CAD build for the part. Positions are in the model's coordinates, mm. A direction names the side the tool comes from. Round coordinates to 2 decimals unless told otherwise and drop trailing zeros. Loops run counter-clockwise (first coordinate to the right, second up) from the corner with the lowest first, then second, coordinate; pieces in that order, holes last. Notation, with made-up numbers: (82, -39) - (131, -39) arc R13 ccw to (131, -34) - close; hole circle Ø7 at (-14.5, 39.5). An arc over 180 degrees is marked (long way). Use one line per item in the form item = value.
from build123d import *

# Parameters (mm, degrees)
SKETCH2_R           = 2.286
BOSS_EXTRUDE1_DEPTH = 5.08
FILLET1_R           = 2.54
FILLET2_R           = 0.635
SKETCH3_W           = 3.81
SKETCH3_H           = 1.905
CUT_EXTRUDE1_DEPTH  = 6.08


with BuildPart() as part:
    # Sketch2 → Boss-Extrude1 (new body)
    with BuildSketch(Plane.XY):
        with BuildLine():
            ThreePointArc((20.32, -7.62), (9.895271997, -11.792143987), (-1.27, -12.983127033))
            Line((-1.27, -12.983127033), (-1.27, -3.81))
            Line((-1.27, -3.81), (20.32, -3.81))
            Line((20.32, -3.81), (20.32, 3.81))
            Line((20.32, 3.81), (-5.08, 3.81))
            Line((-5.08, 3.81), (-5.08, -19.05))
            Line((-5.08, -19.05), (20.32, -19.05))
            Line((20.32, -19.05), (20.32, -7.62))
        make_face()
        Circle(SKETCH2_R, mode=Mode.SUBTRACT)
    extrude(amount=BOSS_EXTRUDE1_DEPTH)

    # Fillet1
    fillet1_edges = [part.edges().sort_by_distance(p)[0] for p in [
        (-5.08, 3.81, 2.54),
        (20.32, 3.81, 2.54),
        (20.32, -3.81, 2.54),
        (-1.27, -3.81, 2.54),
        (20.32, -19.05, 2.54),
        (-5.08, -19.05, 2.54),
    ]]
    fillet(fillet1_edges, radius=FILLET1_R)

    # Fillet2
    fillet2_edges = [part.edges().sort_by_distance(p)[0] for p in [
        (20.32, -7.62, 2.54),
    ]]
    fillet(fillet2_edges, radius=FILLET2_R)

    # Sketch3 → Cut-Extrude1 (cut, through all)
    with BuildSketch(Plane.XY.offset(5.08)):
        with Locations((5.715, 2.8575)):
            Rectangle(SKETCH3_W, SKETCH3_H)
        with Locations((5.715, -2.8575)):
            Rectangle(SKETCH3_W, SKETCH3_H)
        with Locations((14.605, 2.8575)):
            Rectangle(SKETCH3_W, SKETCH3_H)
        with Locations((14.605, -2.8575)):
            Rectangle(SKETCH3_W, SKETCH3_H)
    extrude(amount=-CUT_EXTRUDE1_DEPTH, mode=Mode.SUBTRACT)


solid = part.part
1) Flat gauge pins, fed straight in: pin 1 (1 mm diameter, centred on y = 3, z = 3, fed in from +X); pin 2 (1 mm diameter, centred on y = -2.5, z = 2, fed in from +X); pin 3 (1.1 mm diameter, centred on x = 14.5, z = 1.5, fed in from +Y) (3 decimals); pin 4 (4 mm diameter, centred on x = 13.5, y = -3, fed in from +Z). Where does each tip first touch, or does it go through?
Report:
pin_1 = 20
pin_2 = 20.21
pin_3 = 1.905
pin_4 = 5.08
2) Drill centre lines: probe 1 along Y at (x, z) = (0, 1.8); probe 2 along Y at (x, z) = (3.75, 2.35); probe 3 along X at (y, z) = (-8, 2.6). Where is each one in solid material? Low to high.
Report:
probe_1 = -19.05 to -13, -4.15 to -2.29, 2.29 to 3.81
probe_2 = -19.05 to -12.83, -3.81 to 3.81
probe_3 = -5.08 to -1.27
3) Two-plate mould, pull along Y, no slides. Class faces 1 (the cylindrical face through (-4.316, -18.326, 2.576)), 2 (the flat face through (7, -13, 5.08)), 3 (the flat face through (16.51, -3, 3)): +Y half, -Y half, draft (parallel to the pull), parting line (faces both ways), or undercut.
Report:
face_1 = -Y half
face_2 = draft
face_3 = undercut
4) Tool access for faces 4 (the flat face through (10, -3.81, 3)), 5 (the flat face through (16.51, 3, 3)), 6 (the flat face through (17, 3.81, 3)), 7 (the flat face through (15, -1.905, 3)): list every direction of +Z, -Z, +X, -X, +Y, -Y with a clear straight run to the whole face (end or side of a thin tool).
Report:
face_4 = +Z, -Z, +X
face_5 = +Z, -Z, +Y
face_6 = +Z, -Z, +X, -X, +Y
face_7 = +Z, -Z
5) Slice it at A-A (y = 0). Write the cut outline in (x, z).
Report:
outline = (-5.08, 0) - (-2.29, 0) - (-2.29, 5.08) - (-5.08, 5.08) - close; (2.29, 0) - (20.32, 0) - (20.32, 5.08) - (2.29, 5.08) - close
6) Slice it at D-D (x = 9.25). Write the cut outline in (y, z), plus the area to 3 significant figures.
Report:
outline = (-19.05, 0) - (-11.95, 0) - (-11.95, 5.08) - (-19.05, 5.08) - close; (-3.81, 0) - (3.81, 0) - (3.81, 5.08) - (-3.81, 5.08) - close
area = 74.8 mm^2
7) Slice it at C-C (x = 0). Write the cut outline in (y, z).
Report:
outline = (-19.05, 0) - (-13, 0) - (-13, 5.08) - (-19.05, 5.08) - close; (-4.15, 0) - (-2.29, 0) - (-2.29, 5.08) - (-4.15, 5.08) - close; (2.29, 0) - (3.81, 0) - (3.81, 5.08) - (2.29, 5.08) - close
